Design review of the part built by this model. Coordinates are the model's own, in mm. A direction names the side the tool comes from. Coordinates: 2 decimals unless noted, no trailing zeros. Loops run counter-clockwise (first coordinate to the right, second up) from the corner with the lowest first, then second, coordinate; pieces in that order, holes last.
Autodesk Inventor part; units mm, degrees
ref_plane "YZ Plane" through (0, 0, 0) normal (1, 0, 0) x (0, 1, 0)
ref_plane "XZ Plane" through (0, 0, 0) normal (0, 1, 0) x (-1, 0, 0)
ref_plane "XY Plane" through (0, 0, 0) normal (0, 0, 1) x (1, 0, 0)
sketch "Sketch2" plane through (0, 0, 0) normal (0, 1, 0) x (-1, 0, 0)
  line L0 (0, 0) -> (-59, 0)
  line L1 (-59, 0) -> (-59, 78)
  line L2 (-59, 78) -> (0, 78)
  line L3 (0, 78) -> (0, 0)
  dimension "d0" = 59
  dimension "d1" = 78
extrude "Extrusion1" add sketch "Sketch2" along normal blind 25
shell "Shell1" thickness 3 removed faces 1 at (39.3333, 25, 52)
sketch "Sketch4" plane through (59, 0, 0) normal (0, 0, -1) x (-1, 0, 0)
  point P0 (59, 0)
sketch "Sketch5" plane through (3, 3, 3) normal (0, 0, 1) x (1, 0, 0)
  line L0 (0, 0) -> (0, 22)
  line L1 (0, 22) -> (53, 22)
  line L2 (0, 0) -> (53, 0)
  line L3 (53, 0) -> (53, 22)
  line L4 (53, 22) -> (0, 22)
  line L5 (0, 22) -> (0, 0)
  point P0 (-3, -3)
extrude "Extrusion3" cut sketch "Sketch5" against normal blind 10
sketch "Sketch6" plane through (0, 0, 0) normal (-1, 0, 0) x (0, 0, 1)
  line L0 (4.5, 21.5) -> (30.5, 21.5)
  line L1 (30.5, 21.5) -> (30.5, 17.5)
  line L2 (30.5, 17.5) -> (4.5, 17.5)
  line L3 (4.5, 17.5) -> (4.5, 21.5)
  line L4 (0, 0) -> (0, 25)
  line L5 (0, 0) -> (78, 0)
  dimension "d19" = 26
  dimension "d20" = 4
  dimension "d21" = 4.5
  dimension "d22" = 17.5
sketch "Sketch7" plane through (59, 0, 78) normal (1, 0, 0) x (0, 0, -1)
  line L0 (0, 0) -> (78, 0)
  line L1 (0, 25) -> (78, 25)
  line L2 (78, 25) -> (78, 0)
  line L3 (78, 0) -> (0, 0)
  line L4 (0, 0) -> (0, 25)
extrude "Extrusion5" add sketch "Sketch7" along normal blind 3
extrude "Extrusion6" cut sketch "Sketch6" against normal through all
properties part number "arduino array box v05"
Q1. The part is to be moulded in two halves that separate along Z. For faces 1 (the flat face through (59, 17.5, 18)), 2 (the flat face through (1, 21.5, 17)), 3 (the flat face through (31, 12, 78)), 4 (the flat face through (33, 2, 0)), say which applies: pulls with the +Z half, pulls with the -Z half, needs draft (parallel to the pull), parting line crosses it, or undercut.
Q2. Take a section at B-B, the plane y = 19.75. Write out the cut boundary in (x, z), then the cut area to 3 significant figures.
Q3. Take a section at D-D, the plane x = 21. Write out the cut boundary in (y, z).
Q4. Take a section at C-C, the plane x = 58.5. Write out the cut boundary in (y, z).
Q5. For line 1 (X direction, y = 8.25, z = 39); line 2 (Z direction, x = 9, y = 3.5); line 3 (Y direction, x = 37.5, z = 62), list the stretches that pass through material, from the lowest coordinate up.
Q6. Take a section at A-A, the plane z = 11.5. Write out the cut boundary in (x, y), then the cut area to 3 significant figures.
Q7. Machinability: for faces 5 (the flat face through (58, 25, 45)), 6 (the flat face through (1, 20, 30.5)), 7 (the flat face through (56, 14, 38)), which of the approach directions +Z, -Z, +X, -X, +Y, -Y give a long, thin tool a straight path to every point of the face, cutting with its end or side? Answer none if there is none.
Q8. Clearance check with flat-ended pins moving along their axes: pin 1 Ø5 at (x, z) = (46, 40.5) entering from +Y; pin 2 Ø3 at (x, y) = (40, 20) entering from -Z. State where each tip first meets the part, or that it passes through.
Entries:
1. face 1: undercut
1. face 2: undercut
1. face 3: pulls with the +Z half
1. face 4: pulls with the -Z half
2. outline: (0, 0) - (3, 0) - (3, 4.5) - (0, 4.5) - close; (0, 30.5) - (3, 30.5) - (3, 75) - (56, 75) - (56, 30.5) - (62, 30.5) - (62, 78) - (0, 78) - close; (56, 0) - (62, 0) - (62, 4.5) - (56, 4.5) - close
2. area: 627 mm2
3. outline: (0, 0) - (3, 0) - (3, 75) - (25, 75) - (25, 78) - (0, 78) - close
4. outline: (0, 0) - (25, 0) - (25, 78) - (0, 78) - close; hole (17.5, 4.5) - (21.5, 4.5) - (21.5, 30.5) - (17.5, 30.5) - close
5. line 1: x = 0 to 3, 56 to 62
5. line 2: z = 75 to 78
5. line 3: y = 0 to 3
6. outline: (0, 0) - (62, 0) - (62, 17.5) - (56, 17.5) - (56, 3) - (3, 3) - (3, 17.5) - (0, 17.5) - close; (0, 21.5) - (3, 21.5) - (3, 25) - (0, 25) - close; (56, 21.5) - (62, 21.5) - (62, 25) - (56, 25) - close
6. area: 348 mm2
7. face 5: +Z, -Z, +X, -X, +Y
7. face 6: +X, -X
7. face 7: -Z, +Y
8. pin 1: stops at y = 3
8. pin 2: stops at z = 75
